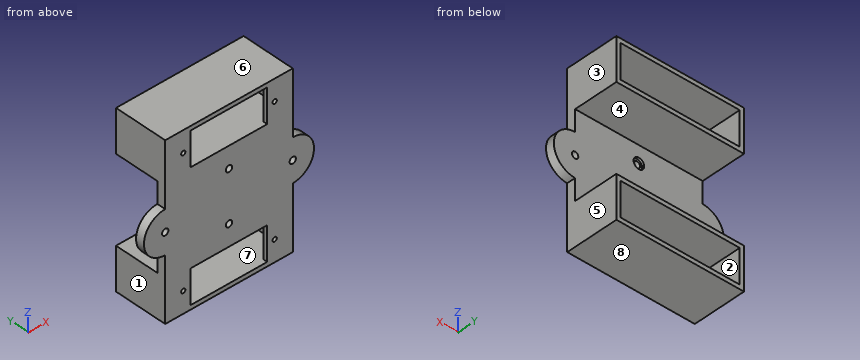
```python
from build123d import *

# Parameters (mm, degrees)
SKETCH1_R           = 1.5
SKETCH1_R_2         = 1
SKETCH1_W           = 36
SKETCH1_H           = 16
BOSS_EXTRUDE1_DEPTH = 4
SKETCH3_W           = 60
SKETCH3_H           = 20
SKETCH3_W_2         = 56
SKETCH3_H_2         = 16
BOSS_EXTRUDE2_DEPTH = 21
SKETCH4_R           = 2.5
CUT_EXTRUDE1_DEPTH  = 1
SKETCH5_W           = 56
SKETCH5_H           = 16
CUT_EXTRUDE2_DEPTH  = 23


with BuildPart() as part:
    # Sketch1 → Boss-Extrude1 (new body)
    with BuildSketch(Plane(origin=(0, 0, 0), x_dir=(1, 0, 0), z_dir=(0, 1, 0))):
        with BuildLine():
            Line((-30, -40), (30, -40))
            Line((30, -40), (30, -10))
            ThreePointArc((30, -10), (40, 0), (30, 10))
            Line((30, 10), (30, 40))
            Line((30, 40), (-30, 40))
            Line((-30, 40), (-30, 10))
            ThreePointArc((-30, 10), (-40, 0), (-30, -10))
            Line((-30, -10), (-30, -40))
        make_face()
        with Locations(Location((30, 0, 0), (0, 0, 90))):
            Circle(SKETCH1_R, mode=Mode.SUBTRACT)
        with Locations(Location((-30, 0, 0), (0, 0, 270))):
            Circle(SKETCH1_R, mode=Mode.SUBTRACT)
        with Locations(Location((0, 12, 0), (0, 0, 270))):
            Circle(SKETCH1_R, mode=Mode.SUBTRACT)
        with Locations(Location((0, -12, 0), (0, 0, 90))):
            Circle(SKETCH1_R, mode=Mode.SUBTRACT)
        with Locations(Location((-21.5, 30, 0), (0, 0, 270))):
            Circle(SKETCH1_R_2, mode=Mode.SUBTRACT)
        with Locations(Location((21.5, 30, 0), (0, 0, 90))):
            Circle(SKETCH1_R_2, mode=Mode.SUBTRACT)
        with Locations(Location((21.5, -30, 0), (0, 0, 270))):
            Circle(SKETCH1_R_2, mode=Mode.SUBTRACT)
        with Locations(Location((-21.5, -30, 0), (0, 0, 90))):
            Circle(SKETCH1_R_2, mode=Mode.SUBTRACT)
        with Locations((0, -30)):
            Rectangle(SKETCH1_W, SKETCH1_H, mode=Mode.SUBTRACT)
        with Locations((0, 30)):
            Rectangle(SKETCH1_W, SKETCH1_H, mode=Mode.SUBTRACT)
    extrude(amount=BOSS_EXTRUDE1_DEPTH)

    # Sketch3 → Boss-Extrude2 (add)
    # profile 1 of 2: a face of its own
    with BuildSketch(Plane(origin=(0, 4, 0), x_dir=(1, 0, 0), z_dir=(0, 1, 0))):
        with Locations((0, 30)):
            Rectangle(SKETCH3_W, SKETCH3_H)
        with Locations((0, 30)):
            Rectangle(SKETCH3_W_2, SKETCH3_H_2, mode=Mode.SUBTRACT)
    # profile 2 of 2: a face of its own
    with BuildSketch(Plane(origin=(0, 4, 0), x_dir=(1, 0, 0), z_dir=(0, 1, 0))):
        with Locations((0, -30)):
            Rectangle(SKETCH3_W, SKETCH3_H)
        with Locations((0, -30)):
            Rectangle(SKETCH3_W_2, SKETCH3_H_2, mode=Mode.SUBTRACT)
    extrude(amount=BOSS_EXTRUDE2_DEPTH)

    # Sketch4 → Cut-Extrude1 (cut)
    with BuildSketch(Plane(origin=(0, 4, 0), x_dir=(1, 0, 0), z_dir=(0, 1, 0))):
        with Locations(Location((0, 12, 0), (0, 0, 270))):
            Circle(SKETCH4_R)
        with Locations(Location((0, -12, 0), (0, 0, 90))):
            Circle(SKETCH4_R)
    extrude(amount=-CUT_EXTRUDE1_DEPTH, mode=Mode.SUBTRACT)

    # Sketch5 → Cut-Extrude2 (cut)
    with BuildSketch(Plane(origin=(0, 25, 0), x_dir=(1, 0, 0), z_dir=(0, 1, 0))):
        with Locations((0, 30)):
            Rectangle(SKETCH5_W, SKETCH5_H)
    cut_extrude2 = extrude(amount=-CUT_EXTRUDE2_DEPTH, mode=Mode.SUBTRACT)

    # Mirror1: Cut-Extrude2 across plane
    add(cut_extrude2.mirror(Plane.XY), mode=Mode.SUBTRACT)


solid = part.part
```
Source: CAD feature listing. Evaluate the final solid. Frame: model axes, mm. Face numbers are marked on the shaded views. A direction names the side the tool comes from. Round coordinates to 2 decimals unless told otherwise and drop trailing zeros. Order: outer loops, then holes, each group sorted by start corner. A loop starts at its lowest first (then second) coordinate and runs counter-clockwise, first axis right, second up. Notation, with made-up numbers: (50, -17.5) -> (95, -17.5) arc R22 cw to (95, 8.5) -> close; hole circle Ø1 at (-4, 37.25). An arc over 180 degrees is marked (long way). One line per item, written item: value. Start each with the question number.
Q1. Material intervals for probe 1 along Z at (x, y) = (-23.5, 23.5); probe 2 along X at (y, z) = (1.2, -30); probe 3 along Z at (x, y) = (-13, 3.75), sorted ascending.
Q2. Section query D-D (z = 12). Return the cut outline in (x, y), plus the area to 3 significant figures.
Q3. Section query A-A (y = 8.5). Return the cut outline in (x, z).
Q4. Pin query (flat end, axial travel): pin 1 (4 mm diameter, centred on y = 10.5, z = 21.5, fed in from +X); pin 2 (3 mm diameter, centred on x = -23.5, z = -31.5, fed in from +Y); pin 3 (8 mm diameter, centred on y = 6, z = 22, fed in from -X). Return the tip coordinate at first contact, or that it passes through.
Q5. Access query for the marked faces 1, 2, 3, 4 and 5. Directions: +Z, -Z, +X, -X, +Y, -Y. A direction counts if a zero-diameter tool reaches every point of the face in a straight line with its end or side. Return the directions, or none.
Q6. Section query B-B (z = -30). Return the cut outline in (x, y).
Q7. Draft query along Z for the marked faces 6, 7 and 8. Return one class per face: pulls with the +Z half, pulls with the -Z half, needs draft (parallel to the pull), parting line crosses it, or undercut.
Q8. Section query C-C (x = -21.5). Return the cut outline in (y, z), plus the area to 3 significant figures.
Findings below:
1. probe 1: -40 to -38, -22 to -20, 20 to 22, 38 to 40
1. probe 2: -30 to -22.5, -20.5 to -18, 18 to 20.5, 22.5 to 30
1. probe 3: -40 to -38, -22 to 22, 38 to 40
2. outline: (-30, 0) -> (-1.5, 0) -> (-1.5, 3) -> (-2.5, 3) -> (-2.5, 4) -> (-30, 4) -> close; (1.5, 0) -> (30, 0) -> (30, 4) -> (2.5, 4) -> (2.5, 3) -> (1.5, 3) -> close
2. area: 226 mm²
3. outline: (-30, -40) -> (30, -40) -> (30, -20) -> (-30, -20) -> close; (-30, 20) -> (30, 20) -> (30, 40) -> (-30, 40) -> close; hole (-28, -38) -> (28, -38) -> (28, -22) -> (-28, -22) -> close; hole (-28, 22) -> (28, 22) -> (28, 38) -> (-28, 38) -> close
4. pin 1: x = 30
4. pin 2: y = 2
4. pin 3: x = -30
5. face 1: -Z, -X, +Y, -Y
5. face 2: +Y
5. face 3: +Z, +X, +Y, -Y
5. face 4: +X, -X, +Y
5. face 5: -Z, +X, +Y, -Y
6. outline: (-30, 0) -> (-22.5, 0) -> (-22.5, 2) -> (-28, 2) -> (-28, 25) -> (-30, 25) -> close; (-20.5, 0) -> (-18, 0) -> (-18, 2) -> (-20.5, 2) -> close; (18, 0) -> (20.5, 0) -> (20.5, 2) -> (18, 2) -> close; (22.5, 0) -> (30, 0) -> (30, 25) -> (28, 25) -> (28, 2) -> (22.5, 2) -> close
7. face 6: pulls with the +Z half
7. face 7: undercut
7. face 8: pulls with the -Z half
8. outline: (0, -40) -> (25, -40) -> (25, -38) -> (2, -38) -> (2, -31) -> (0, -31) -> close; (0, -29) -> (2, -29) -> (2, -22) -> (25, -22) -> (25, -20) -> (4, -20) -> (4, 20) -> (25, 20) -> (25, 22) -> (2, 22) -> (2, 29) -> (0, 29) -> close; (0, 31) -> (2, 31) -> (2, 38) -> (25, 38) -> (25, 40) -> (0, 40) -> close
8. area: 416 mm²
